Read the model definition and answer for the solid it produces. Units are mm, in the model's axes. A direction names the side the tool comes from. Coordinates: 2 decimals unless noted, no trailing zeros. Write each loop counter-clockwise with the first axis right and the second up, starting at its lowest first coordinate (ties: lowest second). Pieces come first, ordered by that corner, then holes.
Item 1: Section A-A (x = -14) is taken. Give the vertices of the cut face in (y, z), then the cut area to 3 significant figures.
Item 2: Straight lines are drawn through the part: probe 1 along X at (y, z) = (5.25, -6) (3 decimals); probe 2 along Z at (x, y) = (-16.75, 1); probe 3 along X at (y, z) = (-5.5, -3). For each, find the intervals that lie inside material, in ascending order.
Item 3: Determine the mould class of faces 3 (the face through (-18.263, -5.796, -7.559)), 4 (the face through (-5.27, -1.25, -0.28)), 5 (the face through (-8.014, 0.584, 1.855)) for opening direction X: released by +X, released by -X, zero draft, split by the parting line, or undercut.
Item 4: Section B-B (x = -7.75) is taken. Give the vertices of the cut face in (y, z).
Item 5: Each of these flat-tipped pins is pushed along its axis until it touches: P1, Ø2, axis at x = -14, z = 4.5, coming from the -Y side; P2, Ø2, axis at x = -14.5, z = 6, coming from the -Y side; P3, Ø2, axis at x = -11, y = -1.5, coming from the +Z side; P4, Ø1, axis at x = -15.5, y = -0.5, coming from the -Z side. Where does it stop, or does it pass through?
Item 6: A tool of negligible diameter and unlimited length cuts with its end or side. For faces 1 (the face through (-17.145, 7, -3)), 2 (the face through (-19.05, 0, 0)), from which of +Z, -Z, +X, -X, +Y, -Y can it reach the whole face along a straight path? Write none if from no direction.
from build123d import *

# Parameters (mm, degrees)
F2_R = 0.635
F3_R = 0.3175


with BuildPart() as f1:
    # F0 (on Front) → F1 (revolve)
    with BuildSketch(Plane.XZ):
        with BuildLine():
            Line((-19.05, 0), (0, 0))
            ThreePointArc((0, 0), (-2.225907, 1.668059), (-4.959707, 1.154812))
            Line((-4.959707, 1.154812), (-6.728575, 1.862012))
            Line((-6.728575, 1.862012), (-9.263298, 2.025665))
            ThreePointArc((-9.263298, 2.025665), (-10.728525, 3.331919), (-12.63395, 3.803665))
            Line((-12.63395, 3.803665), (-15.17395, 3.803665))
            Line((-15.17395, 3.803665), (-17.145, 7.064196))
            Line((-17.145, 7.064196), (-17.145, 9.525))
            Line((-17.145, 9.525), (-19.05, 9.525))
            Line((-19.05, 9.525), (-19.05, 0))
        make_face()
    revolve(axis=Axis((-9.525, 0, 0), (-1, 0, 0)))

    # F2
    f2_edges = [f1.edges().sort_by_distance(p)[0] for p in [
        (-17.145, 0, -9.525),
    ]]
    fillet(f2_edges, radius=F2_R)

    # F3
    f3_edges = [f1.edges().sort_by_distance(p)[0] for p in [
        (-19.05, 0, -9.525),
    ]]
    fillet(f3_edges, radius=F3_R)


solid = f1.part
Established:
1. outline: circle Ø7.61 at (0, 0)
1. area: 45.5 mm2
2. probe 1: x = -19.05 to -17.145
2. probe 2: z = -6.33 to 6.33
2. probe 3: x = -19.05 to -16.66
3. face 3: zero draft
3. face 4: undercut
3. face 5: released by +X
4. outline: circle Ø3.86 at (0, 0)
5. P1: stops at y = -1.49
5. P2: passes through
5. P3: stops at z = 3.61
5. P4: stops at z = -5.15
6. face 1: +X
6. face 2: +Z, -Z, -X, +Y, -Y
